Input: part model. Units: mm. Frame: model coordinates. A direction names the side the tool comes from. Coordinates: 2 decimals unless noted, no trailing zeros. Loops run counter-clockwise (first coordinate to the right, second up) from the corner with the lowest first, then second, coordinate; pieces in that order, holes last. Notation, with made-up numbers: (18, -21.75) -> (73, -21.75) arc R20 cw to (73, 17.25) -> close; hole circle Ø8 at (71.25, 6). An arc over 180 degrees is marked (long way). Answer as a JSON object with one key per item and string values.
from build123d import *

# Parameters (mm, degrees)
F0_R     = 15.5702
F0_R_2   = 3.302
F1_DEPTH = 2.286


# Not quite as in the source:
# - a feature names something its author has since deleted; it is built from what else it names


with BuildPart() as f1:
    # F0 (on Right) → F1 (new body)
    with BuildSketch(Plane.YZ):
        with BuildLine():
            Line((-45.1142073236, -26.818738899), (-411.6793204181, -9.9719436831))
            ThreePointArc((-411.6793204181, -9.9719436831), (-433.0208080629, -17.1370033148), (-443.9559804746, -36.8148888401))
            Line((-443.9559804746, -36.8148888401), (-444.9130844184, -43.7378478567))
            ThreePointArc((-444.9130844184, -43.7378478567), (-438.0085876413, -67.9142971029), (-415.4957405146, -79.1100323691))
            Line((-415.4957405146, -79.1100323691), (-326.7930180723, -83.186679455))
            ThreePointArc((-326.7930180723, -83.186679455), (-322.4925045261, -85.1441378233), (-320.7345470438, -89.5299838666))
            Line((-320.7345470438, -89.5299838666), (-320.7345470438, -151.0368096017))
            ThreePointArc((-320.7345470438, -151.0368096017), (-318.8746751043, -155.5269376622), (-314.3845470438, -157.3868096017))
            Line((-314.3845470438, -157.3868096017), (-274.5700470438, -157.3868096017))
            ThreePointArc((-274.5700470438, -157.3868096017), (-270.0799189833, -155.5269376622), (-268.2200470438, -151.0368096017))
            Line((-268.2200470438, -151.0368096017), (-268.2200470438, -92.5271466826))
            ThreePointArc((-268.2200470438, -92.5271466826), (-266.2558930871, -87.9351041649), (-261.5785180723, -86.183842271))
            Line((-261.5785180723, -86.183842271), (-169.4194716536, -90.4193369398))
            ThreePointArc((-169.4194716536, -90.4193369398), (-165.1189581074, -92.3767953082), (-163.3610006251, -96.7626413515))
            Line((-163.3610006251, -96.7626413515), (-163.3610006251, -151.0368096017))
            ThreePointArc((-163.3610006251, -151.0368096017), (-161.5011286857, -155.5269376622), (-157.0110006251, -157.3868096017))
            Line((-157.0110006251, -157.3868096017), (-117.1965006251, -157.3868096017))
            ThreePointArc((-117.1965006251, -157.3868096017), (-112.7063725646, -155.5269376622), (-110.8465006251, -151.0368096017))
            Line((-110.8465006251, -151.0368096017), (-110.8465006251, -99.7598041674))
            ThreePointArc((-110.8465006251, -99.7598041674), (-108.8823466684, -95.1677616497), (-104.2049716536, -93.4164997558))
            Line((-104.2049716536, -93.4164997558), (-32.7059788978, -96.7024886458))
            ThreePointArc((-32.7059788978, -96.7024886458), (-28.3737210787, -98.6934263777), (-26.6481782752, -103.1380627967))
            Line((-26.6481782752, -103.1380627967), (-27.3295071805, -150.0221421965))
            ThreePointArc((-27.3295071805, -150.0221421965), (-25.5028102734, -154.5717983424), (-20.9801775863, -156.4644119358))
            Line((-20.9801775863, -156.4644119358), (17.7761926764, -156.4644119358))
            ThreePointArc((17.7761926764, -156.4644119358), (22.266320737, -154.6045399963), (24.1261926764, -150.1144119358))
            Line((24.1261926764, -150.1144119358), (24.1261926764, -99.3144119358))
            Line((24.1261926764, -99.3144119358), (24.1261926764, -36.0657921419))
            ThreePointArc((24.1261926764, -36.0657921419), (22.3682351942, -31.6799460986), (18.0677216479, -29.7224877302))
            Line((18.0677216479, -29.7224877302), (-45.1142073236, -26.818738899))
        make_face()
        with Locations((-410.0968120394, -44.7014163277)):
            Circle(F0_R, mode=Mode.SUBTRACT)
        with Locations((-305.1785570708, -49.5233055166)):
            Circle(F0_R, mode=Mode.SUBTRACT)
        with Locations((-200.2603021023, -54.3451947055)):
            Circle(F0_R, mode=Mode.SUBTRACT)
        with Locations((-95.3420471337, -59.1670838944)):
            Circle(F0_R, mode=Mode.SUBTRACT)
        with Locations((-10.4940073236, -63.0665754174)):
            Circle(F0_R, mode=Mode.SUBTRACT)
        with BuildLine():
            Line((-45.1142073236, 51.7922245826), (-45.1142073236, -26.818738899))
            Line((-45.1142073236, -26.818738899), (18.0677216479, -29.7224877302))
            Line((18.0677216479, -29.7224877302), (24.1261926764, -30.000926177))
            Line((24.1261926764, -30.000926177), (24.1261926764, 51.7922245826))
            ThreePointArc((24.1261926764, 51.7922245826), (15.0053806853, 73.8118125915), (-7.0142073236, 82.9326245826))
            Line((-7.0142073236, 82.9326245826), (-13.9738073236, 82.9326245826))
            ThreePointArc((-13.9738073236, 82.9326245826), (-35.9933953324, 73.8118125915), (-45.1142073236, 51.7922245826))
        make_face()
        with Locations((-10.4940073236, 15.6400269167)):
            Circle(F0_R_2, mode=Mode.SUBTRACT)
        with Locations((-10.4940073236, 41.9624245826)):
            Circle(F0_R, mode=Mode.SUBTRACT)
        with Locations((-10.4940073236, 66.4400269167)):
            Circle(F0_R_2, mode=Mode.SUBTRACT)
        with BuildLine():
            Line((24.1261926764, -30.000926177), (18.0677216479, -29.7224877302))
            ThreePointArc((18.0677216479, -29.7224877302), (22.3682351942, -31.6799460986), (24.1261926764, -36.0657921419))
            Line((24.1261926764, -36.0657921419), (24.1261926764, -30.000926177))
        make_face()
    extrude(amount=F1_DEPTH)


solid = f1.part
1. Access query for faces 4 (the face through (1.127, -320.734, -48.839)), 5 (the face through (1.127, -225.831, -18.513)). Directions: +Z, -Z, +X, -X, +Y, -Y. A direction counts if a zero-diameter tool reaches every point of the face in a straight line with its end or side. Return the directions, or none.
Reply:
{"face 4": "+X, -X", "face 5": "+Z, +X, -X"}
2. Line query: line 1 along Y through (x, z) = (1.15, -103.5); line 2 along Y through (x, z) = (0.8, -112.5); line 3 along Z through (x, y) = (1.9, -24). Output: solid intervals per line, ascending.
Reply:
{"line 1": "y = -320.73 to -268.22, -163.36 to -110.85, -26.65 to 24.13", "line 2": "y = -320.73 to -268.22, -163.36 to -110.85, -26.78 to 24.13", "line 3": "z = -155.7 to -70.81, -55.32 to 34.22, 49.71 to 81.27"}
3. Section query C-C (x = 0.7). Count the separate pieces of the cut face and the enclosed holes in it, plus the area to 3 significant figures.
Reply:
{"separate pieces": "1", "enclosed holes": "8", "area": "45,000 mm2"}
4. Mould query, pull axis Z, two halves, no side actions, for faces 1 (the face through (1.13, -2.12, -49.94)), 2 (the face through (1.127, 15.246, 73.568)), 3 (the face through (2.286, -159, -63)). Classes: pulls with the +Z half, pulls with the -Z half, needs draft (parallel to the pull), parting line crosses it, or undercut.
Reply:
{"face 1": "undercut", "face 2": "pulls with the +Z half", "face 3": "needs draft"}
5. Section query B-B (y = -305.5). Return loops of the section in (x, z), plus the area to 3 significant figures.
Reply:
{"outline": "(0, -157.39) -> (2.29, -157.39) -> (2.29, -65.09) -> (0, -65.09) -> close; (0, -33.96) -> (2.29, -33.96) -> (2.29, -14.85) -> (0, -14.85) -> close", "area": "255 mm2"}
6. Section query D-D (y = -242.5). Return loops of the section in (x, z), plus the area to 3 significant figures.
Reply:
{"outline": "(0, -87.06) -> (2.29, -87.06) -> (2.29, -17.75) -> (0, -17.75) -> close", "area": "158 mm2"}
7. Section query A-A (z = -124.5). Return loops of the section in (x, y), plus the area to 3 significant figures.
Reply:
{"outline": "(0, -320.73) -> (2.29, -320.73) -> (2.29, -268.22) -> (0, -268.22) -> close; (0, -163.36) -> (2.29, -163.36) -> (2.29, -110.85) -> (0, -110.85) -> close; (0, -26.96) -> (2.29, -26.96) -> (2.29, 24.13) -> (0, 24.13) -> close", "area": "357 mm2"}
8. Pin query (flat end, axial travel): P1, Ø0.7, axis at x = 1.5, y = -0.5, coming from the -Z side; P2, Ø1.1, axis at x = 1, z = -1, coming from the -Y side; P3, Ø25, axis at y = -95.34, z = -59.17, coming from the -X side; P4, Ø1.1, axis at x = 0.5, z = -133, coming from the -Y side. Return the tip coordinate at first contact, or that it passes through.
Reply:
{"P1": "stops at z = -156.46", "P2": "stops at y = -45.11", "P3": "passes through", "P4": "stops at y = -320.73"}
